Could you check a few things on this model? Use its own coordinates, in mm. Face numbers are marked on the shaded views. A direction names the side the tool comes from. Round coordinates to 2 decimals unless told otherwise and drop trailing zeros. Loops run counter-clockwise (first coordinate to the right, second up) from the corner with the lowest first, then second, coordinate; pieces in that order, holes last. Notation, with made-up numbers: (5, 7) -> (61, 7) arc R34 cw to (61, 41) -> close; hole circle Ø4 at (25, -25.75). An arc over 180 degrees is marked (long way). One line per item, written item: value.
```python
from build123d import *

# Parameters (mm, degrees)
BOSS_EXTRUDE1_DEPTH       = 15.875
SHELL1_T                  = -8.89
F_4_40_TAPPED_HOLE1_D     = 2.2606
F_4_40_TAPPED_HOLE1_DEPTH = 7.62
F_4_40_TAPPED_HOLE1_TIP   = 0.679153
SKETCH6_W                 = 180.34
SKETCH6_H                 = 6.35
BOSS_EXTRUDE2_DEPTH       = 177.8
SKETCH7_W                 = 127
SKETCH7_H                 = 95.25
CUT_EXTRUDE2_DEPTH        = 7.62
CUT_EXTRUDE3_REACH        = 256.155


with BuildPart() as part:
    # Sketch1 → Boss-Extrude1 (new, symmetric)
    with BuildSketch(Plane.XY):
        with BuildLine():
            ThreePointArc((0, -50.8), (-35.921024, -35.921024), (-50.8, 0))
            Line((-50.8, 0), (-67.31, 0))
            Line((-67.31, 0), (-67.31, -128.524))
            Line((-67.31, -128.524), (-88.9, -128.524))
            Line((-88.9, -128.524), (-88.9, -134.874))
            Line((-88.9, -134.874), (0, -134.874))
            Line((0, -134.874), (0, -50.8))
        make_face()
        with BuildLine():
            ThreePointArc((50.8, 0), (35.921024, -35.921024), (0, -50.8))
            Line((0, -50.8), (0, -134.874))
            Line((0, -134.874), (88.9, -134.874))
            Line((88.9, -134.874), (88.9, -128.524))
            Line((88.9, -128.524), (67.31, -128.524))
            Line((67.31, -128.524), (67.31, 0))
            Line((67.31, 0), (50.8, 0))
        make_face()
    extrude(amount=BOSS_EXTRUDE1_DEPTH, both=True)

    # Shell1
    shell1_openings = [part.faces().sort_by_distance(p)[0] for p in [
        (0, -81.597488, 15.875),
        (0, -81.597488, -15.875),
    ]]
    offset(amount=SHELL1_T, openings=shell1_openings)

    # #4-40 Tapped Hole1
    with Locations(Plane(origin=(0, 0, 0), x_dir=(1, 0, 0), z_dir=(0, 1, 0))):
        with Locations((-57.658, 5.715), (-57.658, -6.985), (57.658, -6.985), (57.658, 5.715)):
            Hole(F_4_40_TAPPED_HOLE1_D / 2, depth=F_4_40_TAPPED_HOLE1_DEPTH)
            with Locations((0, 0, -(F_4_40_TAPPED_HOLE1_DEPTH + F_4_40_TAPPED_HOLE1_TIP / 2))):  # 118° drill point
                Cone(0, F_4_40_TAPPED_HOLE1_D / 2, F_4_40_TAPPED_HOLE1_TIP, mode=Mode.SUBTRACT)

    # Sketch6 → Boss-Extrude2 (add)
    with BuildSketch(Plane(origin=(88.9, 0, 0), x_dir=(0, 0, -1), z_dir=(1, 0, 0))):
        with Locations((106.045, -131.699)):
            Rectangle(SKETCH6_W, SKETCH6_H)
    extrude(amount=-BOSS_EXTRUDE2_DEPTH)

    # Sketch7 → Cut-Extrude2 (cut)
    with BuildSketch(Plane.XZ.offset(134.874)):
        with Locations((0, -69.85)):
            Rectangle(SKETCH7_W, SKETCH7_H)
    extrude(amount=-CUT_EXTRUDE2_DEPTH, mode=Mode.SUBTRACT)

    # Sketch8 → Cut-Extrude3 (cut, up to next)
    with BuildSketch(Plane.XZ.offset(134.874), mode=Mode.PRIVATE) as cut_extrude3_sk1:
        with BuildLine():
            ThreePointArc((72.39, -1.27), (73.505923, -3.964077), (76.2, -5.08))
            Line((76.2, -5.08), (76.2, -1.27))
            Line((76.2, -1.27), (72.39, -1.27))
        make_face()
    cut_extrude3_tool1 = extrude(cut_extrude3_sk1.sketch, amount=-CUT_EXTRUDE3_REACH, mode=Mode.PRIVATE) & part.part
    # Sketch8 → Cut-Extrude3 (cut, up to next)
    with BuildSketch(Plane.XZ.offset(134.874), mode=Mode.PRIVATE) as cut_extrude3_sk2:
        with BuildLine():
            Line((76.2, -1.27), (76.2, -5.08))
            ThreePointArc((76.2, -5.08), (78.894077, -3.964077), (80.01, -1.27))
            ThreePointArc((80.01, -1.27), (76.2, 2.54), (72.39, -1.27))
            Line((72.39, -1.27), (76.2, -1.27))
        make_face()
    cut_extrude3_tool2 = extrude(cut_extrude3_sk2.sketch, amount=-CUT_EXTRUDE3_REACH, mode=Mode.PRIVATE) & part.part
    # Sketch8 → Cut-Extrude3 (cut, up to next)
    with BuildSketch(Plane.XZ.offset(134.874), mode=Mode.PRIVATE) as cut_extrude3_sk3:
        with BuildLine():
            ThreePointArc((72.39, -1.27), (73.505923, -3.964077), (76.2, -5.08))
            Line((76.2, -5.08), (76.2, -1.27))
            Line((76.2, -1.27), (72.39, -1.27))
        make_face()
    cut_extrude3_tool3 = extrude(cut_extrude3_sk3.sketch, amount=-CUT_EXTRUDE3_REACH, mode=Mode.PRIVATE) & part.part
    # Sketch8 → Cut-Extrude3 (cut, up to next)
    with BuildSketch(Plane.XZ.offset(134.874), mode=Mode.PRIVATE) as cut_extrude3_sk4:
        with BuildLine():
            Line((76.2, -1.27), (76.2, -5.08))
            ThreePointArc((76.2, -5.08), (78.894077, -3.964077), (80.01, -1.27))
            ThreePointArc((80.01, -1.27), (76.2, 2.54), (72.39, -1.27))
            Line((72.39, -1.27), (76.2, -1.27))
        make_face()
    cut_extrude3_tool4 = extrude(cut_extrude3_sk4.sketch, amount=-CUT_EXTRUDE3_REACH, mode=Mode.PRIVATE) & part.part
    # Sketch8 → Cut-Extrude3 (cut, up to next)
    with BuildSketch(Plane.XZ.offset(134.874), mode=Mode.PRIVATE) as cut_extrude3_sk5:
        with BuildLine():
            ThreePointArc((-72.39, -1.27), (-78.894077, 1.424077), (-76.2, -5.08))
            Line((-76.2, -5.08), (-76.2, -1.27))
            Line((-76.2, -1.27), (-72.39, -1.27))
        make_face()
    cut_extrude3_tool5 = extrude(cut_extrude3_sk5.sketch, amount=-CUT_EXTRUDE3_REACH, mode=Mode.PRIVATE) & part.part
    # Sketch8 → Cut-Extrude3 (cut, up to next)
    with BuildSketch(Plane.XZ.offset(134.874), mode=Mode.PRIVATE) as cut_extrude3_sk6:
        with BuildLine():
            Line((-76.2, -1.27), (-76.2, -5.08))
            ThreePointArc((-76.2, -5.08), (-73.505923, -3.964077), (-72.39, -1.27))
            Line((-72.39, -1.27), (-76.2, -1.27))
        make_face()
    cut_extrude3_tool6 = extrude(cut_extrude3_sk6.sketch, amount=-CUT_EXTRUDE3_REACH, mode=Mode.PRIVATE) & part.part
    # Sketch8 → Cut-Extrude3 (cut, up to next)
    with BuildSketch(Plane.XZ.offset(134.874), mode=Mode.PRIVATE) as cut_extrude3_sk7:
        with BuildLine():
            ThreePointArc((-72.39, -1.27), (-78.894077, 1.424077), (-76.2, -5.08))
            Line((-76.2, -5.08), (-76.2, -1.27))
            Line((-76.2, -1.27), (-72.39, -1.27))
        make_face()
    cut_extrude3_tool7 = extrude(cut_extrude3_sk7.sketch, amount=-CUT_EXTRUDE3_REACH, mode=Mode.PRIVATE) & part.part
    # Sketch8 → Cut-Extrude3 (cut, up to next)
    with BuildSketch(Plane.XZ.offset(134.874), mode=Mode.PRIVATE) as cut_extrude3_sk8:
        with BuildLine():
            Line((-76.2, -1.27), (-76.2, -5.08))
            ThreePointArc((-76.2, -5.08), (-73.505923, -3.964077), (-72.39, -1.27))
            Line((-72.39, -1.27), (-76.2, -1.27))
        make_face()
    cut_extrude3_tool8 = extrude(cut_extrude3_sk8.sketch, amount=-CUT_EXTRUDE3_REACH, mode=Mode.PRIVATE) & part.part
    # Sketch8 → Cut-Extrude3 (cut, up to next)
    with BuildSketch(Plane.XZ.offset(134.874), mode=Mode.PRIVATE) as cut_extrude3_sk9:
        with BuildLine():
            ThreePointArc((-76.2, -175.26), (-78.894077, -181.764077), (-72.39, -179.07))
            Line((-72.39, -179.07), (-76.2, -179.07))
            Line((-76.2, -179.07), (-76.2, -175.26))
        make_face()
    cut_extrude3_tool9 = extrude(cut_extrude3_sk9.sketch, amount=-CUT_EXTRUDE3_REACH, mode=Mode.PRIVATE) & part.part
    # Sketch8 → Cut-Extrude3 (cut, up to next)
    with BuildSketch(Plane.XZ.offset(134.874), mode=Mode.PRIVATE) as cut_extrude3_sk10:
        with BuildLine():
            Line((-76.2, -179.07), (-72.39, -179.07))
            ThreePointArc((-72.39, -179.07), (-73.505923, -176.375923), (-76.2, -175.26))
            Line((-76.2, -175.26), (-76.2, -179.07))
        make_face()
    cut_extrude3_tool10 = extrude(cut_extrude3_sk10.sketch, amount=-CUT_EXTRUDE3_REACH, mode=Mode.PRIVATE) & part.part
    # Sketch8 → Cut-Extrude3 (cut, up to next)
    with BuildSketch(Plane.XZ.offset(134.874), mode=Mode.PRIVATE) as cut_extrude3_sk11:
        with BuildLine():
            ThreePointArc((-76.2, -175.26), (-78.894077, -181.764077), (-72.39, -179.07))
            Line((-72.39, -179.07), (-76.2, -179.07))
            Line((-76.2, -179.07), (-76.2, -175.26))
        make_face()
    cut_extrude3_tool11 = extrude(cut_extrude3_sk11.sketch, amount=-CUT_EXTRUDE3_REACH, mode=Mode.PRIVATE) & part.part
    # Sketch8 → Cut-Extrude3 (cut, up to next)
    with BuildSketch(Plane.XZ.offset(134.874), mode=Mode.PRIVATE) as cut_extrude3_sk12:
        with BuildLine():
            Line((-76.2, -179.07), (-72.39, -179.07))
            ThreePointArc((-72.39, -179.07), (-73.505923, -176.375923), (-76.2, -175.26))
            Line((-76.2, -175.26), (-76.2, -179.07))
        make_face()
    cut_extrude3_tool12 = extrude(cut_extrude3_sk12.sketch, amount=-CUT_EXTRUDE3_REACH, mode=Mode.PRIVATE) & part.part
    # Sketch8 → Cut-Extrude3 (cut, up to next)
    with BuildSketch(Plane.XZ.offset(134.874), mode=Mode.PRIVATE) as cut_extrude3_sk13:
        with BuildLine():
            ThreePointArc((76.2, -175.26), (73.505923, -176.375923), (72.39, -179.07))
            Line((72.39, -179.07), (76.2, -179.07))
            Line((76.2, -179.07), (76.2, -175.26))
        make_face()
    cut_extrude3_tool13 = extrude(cut_extrude3_sk13.sketch, amount=-CUT_EXTRUDE3_REACH, mode=Mode.PRIVATE) & part.part
    # Sketch8 → Cut-Extrude3 (cut, up to next)
    with BuildSketch(Plane.XZ.offset(134.874), mode=Mode.PRIVATE) as cut_extrude3_sk14:
        with BuildLine():
            Line((76.2, -179.07), (72.39, -179.07))
            ThreePointArc((72.39, -179.07), (76.2, -182.88), (80.01, -179.07))
            ThreePointArc((80.01, -179.07), (78.894077, -176.375923), (76.2, -175.26))
            Line((76.2, -175.26), (76.2, -179.07))
        make_face()
    cut_extrude3_tool14 = extrude(cut_extrude3_sk14.sketch, amount=-CUT_EXTRUDE3_REACH, mode=Mode.PRIVATE) & part.part
    # Sketch8 → Cut-Extrude3 (cut, up to next)
    with BuildSketch(Plane.XZ.offset(134.874), mode=Mode.PRIVATE) as cut_extrude3_sk15:
        with BuildLine():
            ThreePointArc((76.2, -175.26), (73.505923, -176.375923), (72.39, -179.07))
            Line((72.39, -179.07), (76.2, -179.07))
            Line((76.2, -179.07), (76.2, -175.26))
        make_face()
    cut_extrude3_tool15 = extrude(cut_extrude3_sk15.sketch, amount=-CUT_EXTRUDE3_REACH, mode=Mode.PRIVATE) & part.part
    # Sketch8 → Cut-Extrude3 (cut, up to next)
    with BuildSketch(Plane.XZ.offset(134.874), mode=Mode.PRIVATE) as cut_extrude3_sk16:
        with BuildLine():
            Line((76.2, -179.07), (72.39, -179.07))
            ThreePointArc((72.39, -179.07), (76.2, -182.88), (80.01, -179.07))
            ThreePointArc((80.01, -179.07), (78.894077, -176.375923), (76.2, -175.26))
            Line((76.2, -175.26), (76.2, -179.07))
        make_face()
    cut_extrude3_tool16 = extrude(cut_extrude3_sk16.sketch, amount=-CUT_EXTRUDE3_REACH, mode=Mode.PRIVATE) & part.part
    add(cut_extrude3_tool1.solids().sort_by_distance((74.582986, -134.874, -2.887014))[0], mode=Mode.SUBTRACT)
    add(cut_extrude3_tool2.solids().sort_by_distance((76.739005, -134.874, -0.730995))[0], mode=Mode.SUBTRACT)
    add(cut_extrude3_tool3.solids().sort_by_distance((74.582986, -134.874, -2.887014))[0], mode=Mode.SUBTRACT)
    add(cut_extrude3_tool4.solids().sort_by_distance((76.739005, -134.874, -0.730995))[0], mode=Mode.SUBTRACT)
    add(cut_extrude3_tool5.solids().sort_by_distance((-76.739005, -134.874, -0.730995))[0], mode=Mode.SUBTRACT)
    add(cut_extrude3_tool6.solids().sort_by_distance((-74.582986, -134.874, -2.887014))[0], mode=Mode.SUBTRACT)
    add(cut_extrude3_tool7.solids().sort_by_distance((-76.739005, -134.874, -0.730995))[0], mode=Mode.SUBTRACT)
    add(cut_extrude3_tool8.solids().sort_by_distance((-74.582986, -134.874, -2.887014))[0], mode=Mode.SUBTRACT)
    add(cut_extrude3_tool9.solids().sort_by_distance((-76.739005, -134.874, -179.609005))[0], mode=Mode.SUBTRACT)
    add(cut_extrude3_tool10.solids().sort_by_distance((-74.582986, -134.874, -177.452986))[0], mode=Mode.SUBTRACT)
    add(cut_extrude3_tool11.solids().sort_by_distance((-76.739005, -134.874, -179.609005))[0], mode=Mode.SUBTRACT)
    add(cut_extrude3_tool12.solids().sort_by_distance((-74.582986, -134.874, -177.452986))[0], mode=Mode.SUBTRACT)
    add(cut_extrude3_tool13.solids().sort_by_distance((74.582986, -134.874, -177.452986))[0], mode=Mode.SUBTRACT)
    add(cut_extrude3_tool14.solids().sort_by_distance((76.739005, -134.874, -179.609005))[0], mode=Mode.SUBTRACT)
    add(cut_extrude3_tool15.solids().sort_by_distance((74.582986, -134.874, -177.452986))[0], mode=Mode.SUBTRACT)
    add(cut_extrude3_tool16.solids().sort_by_distance((76.739005, -134.874, -179.609005))[0], mode=Mode.SUBTRACT)


solid = part.part
```
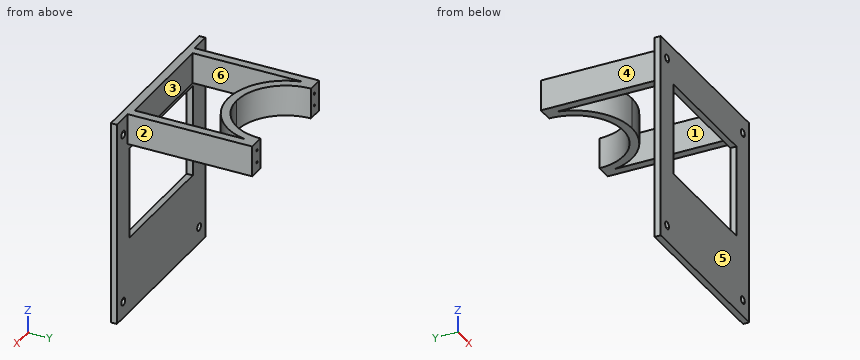
(1) Imagine slicing it at C-C on y = -41.5. Write out the boundary of the cut face in (x, z) (3 decimals).
Results below:
outline: (-67.31, -15.875) -> (-58.42, -15.875) -> (-58.42, 15.875) -> (-67.31, 15.875) -> close; (-42.903, -15.875) -> (-29.298, -15.875) -> (-29.298, 15.875) -> (-42.903, 15.875) -> close; (29.298, -15.875) -> (42.903, -15.875) -> (42.903, 15.875) -> (29.298, 15.875) -> close; (58.42, -15.875) -> (67.31, -15.875) -> (67.31, 15.875) -> (58.42, 15.875) -> close
(2) Please list where these lines run through material, in increasing order: L1, parallel to Z at x = -76, y = -132 (3 decimals); L2, parallel to X at y = -76.5, z = 1.5; L3, parallel to Y at x = 67.5, z = -27.
Results below:
L1: z = -196.215 to -182.875, -175.265 to -5.075, 2.535 to 15.875
L2: x = -67.31 to -58.42, 58.42 to 67.31
L3: y = -134.87 to -128.52
(3) Imagine slicing it at A-A on z = -114. Write out the boundary of the cut face in (x, y).
Results below:
outline: (-88.9, -134.87) -> (-63.5, -134.87) -> (-63.5, -128.52) -> (-88.9, -128.52) -> close; (63.5, -134.87) -> (88.9, -134.87) -> (88.9, -128.52) -> (63.5, -128.52) -> close
(4) Imagine slicing it at B-B on x = -27.5. Write out the boundary of the cut face in (y, z) (3 decimals), then the cut area to 3 significant figures.
Results below:
outline: (-134.874, -196.215) -> (-128.524, -196.215) -> (-128.524, -117.475) -> (-134.874, -117.475) -> close; (-134.874, -22.225) -> (-128.524, -22.225) -> (-128.524, -15.875) -> (-125.984, -15.875) -> (-125.984, 15.875) -> (-134.874, 15.875) -> close; (-52.978, -15.875) -> (-42.713, -15.875) -> (-42.713, 15.875) -> (-52.978, 15.875) -> close
area: 1,150 mm²
(5) Imagine slicing it at D-D on x = 46. Write out the boundary of the cut face in (y, z) (1 decimal).
Results below:
outline: (-134.9, -196.2) -> (-128.5, -196.2) -> (-128.5, -117.5) -> (-134.9, -117.5) -> close; (-134.9, -22.2) -> (-128.5, -22.2) -> (-128.5, -15.9) -> (-126, -15.9) -> (-126, 15.9) -> (-134.9, 15.9) -> close; (-38, -15.9) -> (-21.6, -15.9) -> (-21.6, 15.9) -> (-38, 15.9) -> close
(6) On a 3-axis mill with a long thin cutter (end or side, diameter ignored), from which of +Z, -Z, +X, -X, +Y, -Y can I reach the whole of each face in a straight line? I mean the marked faces 5 and 6. Say none if no direction works.
Results below:
face 5: +Z, -Z, +X, -X, -Y
face 6: +Z, -Z
(7) For pin 1 Ø12 at (x, z) = (-76.2, -1.27) entering from +Y; pin 2 Ø1.4 at (x, z) = (-57.658, 6.985) entering from +Y; pin 3 Ø10 at (y, z) = (-46.5, -20.5) entering from -X; pin 4 Ø3.5 at (x, z) = (57.658, -5.715) entering from +Y, each with a flat end and sliding along its axis, tell me the tip position at first contact or that it passes through.
Results below:
pin 1: stops at y = -128.52
pin 2: stops at y = -7.88
pin 3: stops at x = -67.31
pin 4: stops at y = 0
(8) We'd pull the mould along X, two halves only. Please class the marked faces 1, 2, 3 and 4: +X half, -X half, draft (parallel to the pull), parting line (faces both ways), or undercut.
Results below:
face 1: undercut
face 2: +X half
face 3: undercut
face 4: -X half
